from build123d import *

# Parameters (mm, degrees)
BOSS_EXTRUDE1_DEPTH     = 6.1
SKETCH3_R               = 1.25
CUT_EXTRUDE1_DEPTH      = 28.622092607
MIRROR1_COPY_1_SKETCH_R = 1.25
MIRROR1_COPY_1_DEPTH    = 28.622092607
FILLET1_R               = 1


with BuildPart() as part:
    # Sketch1 → Boss-Extrude1 (new, symmetric)
    with BuildSketch(Plane.XY):
        Polygon((11.6, 7.8), (16.1, 7.8), (16.1, 6.7), (11.6, 6.7), (11.6, -13.8), (-11.6, -13.8), (-11.6, 6.7), (-16.1, 6.7), (-16.1, 7.8), (-11.6, 7.8), (-11.6, 13.8), (11.6, 13.8), align=None)
    extrude(amount=BOSS_EXTRUDE1_DEPTH, both=True)

    # Sketch2 → Revolve1 (revolve)
    with BuildSketch(Plane.XY, mode=Mode.PRIVATE) as revolve1_sk:
        Polygon((-5.6, 18.1), (-8.1, 18.1), (-8.1, 14.8), (-9.430450184, 14.8), (-9.85, 14.3), (-9.85, 13.8), (-5.6, 13.8), align=None)
    revolve(revolve1_sk.sketch.rotate(Axis((-5.6, 13.8, 0), (0, 1, 0)), 270), axis=Axis((-5.6, 13.8, 0), (0, 1, 0)))

    # Sketch3 → Cut-Extrude1 (cut, through all)
    with BuildSketch(Plane(origin=(0, 7.8, 0), x_dir=(1, 0, 0), z_dir=(0, 1, 0))):
        with Locations(Location((14.15, 3.55, 0), (0, 0, 270))):
            Circle(SKETCH3_R)
        with BuildLine():
            Line((16.1, 0), (13.1, 0))
            Line((13.1, 0), (12, 0))
            ThreePointArc((12, 0), (12.322182541, 0.777817459), (13.1, 1.1))
            Line((13.1, 1.1), (16.1, 1.1))
            Line((16.1, 1.1), (16.1, 0))
        make_face()
    cut_extrude1 = extrude(amount=-CUT_EXTRUDE1_DEPTH, mode=Mode.SUBTRACT)

    # Mirror4: Cut-Extrude1 across plane
    add(cut_extrude1.mirror(Plane(origin=(0, 0, 0), x_dir=(0, 0, 1), z_dir=(1, 0, 0))), mode=Mode.SUBTRACT)

    # Mirror1: Cut-Extrude1 across plane
    add(cut_extrude1.mirror(Plane(origin=(16.1, -13.8, 0), x_dir=(1, 0, 0), z_dir=(0, 0, 1))), mode=Mode.SUBTRACT)

    # Mirror1 copy 1 sketch → Mirror1 copy 1 (cut, through all)
    with BuildSketch(Plane(origin=(0, 7.8, 0), x_dir=(-1, 0, 0), z_dir=(0, 1, 0))):
        with Locations(Location((14.15, 3.55, 0), (0, 0, 270))):
            Circle(MIRROR1_COPY_1_SKETCH_R)
        with BuildLine():
            Line((16.1, 0), (13.1, 0))
            Line((13.1, 0), (12, 0))
            ThreePointArc((12, 0), (12.322182541, 0.777817459), (13.1, 1.1))
            Line((13.1, 1.1), (16.1, 1.1))
            Line((16.1, 1.1), (16.1, 0))
        make_face()
    extrude(amount=-MIRROR1_COPY_1_DEPTH, mode=Mode.SUBTRACT)

    # Fillet1
    fillet1_edges = [part.edges().sort_by_distance(p)[0] for p in [
        (-16.1, 7.25, 6.1),
        (16.1, 7.25, -6.1),
        (-16.1, 7.25, -6.1),
        (16.1, 7.25, 6.1),
    ]]
    fillet(fillet1_edges, radius=FILLET1_R)


solid = part.part
Check sheet for the modelled part. Datum: model origin and axes. Units: mm. A direction names the side the tool comes from. Coordinates: 2 decimals unless noted, no trailing zeros. Write each loop counter-clockwise with the first axis right and the second up, starting at its lowest first coordinate (ties: lowest second). Pieces come first, ordered by that corner, then holes.
Item 1: Cross-section at A-A on x = 14.15. Record the boundary of the cut face in (y, z), then the cut area to 3 significant figures.
Numbers:
outline: (6.7, -6.1) - (7.8, -6.1) - (7.8, -4.8) - (6.7, -4.8) - close; (6.7, -2.3) - (7.8, -2.3) - (7.8, -1.1) - (6.7, -1.1) - close; (6.7, 1.1) - (7.8, 1.1) - (7.8, 2.3) - (6.7, 2.3) - close; (6.7, 4.8) - (7.8, 4.8) - (7.8, 6.1) - (6.7, 6.1) - close
area: 5.50 mm2
Item 2: Scan lines: probe 1 along Z at (x, y) = (-14, 7); probe 2 along X at (y, z) = (7.6, -3.55); probe 3 along Y at (x, z) = (-3.5, 1.5). Record each from-to range of solid material in increasing order.
Numbers:
probe 1: z = -6.1 to -4.79, -2.31 to -1.1, 1.1 to 2.31, 4.79 to 6.1
probe 2: x = -16.1 to -15.4, -12.9 to 12.9, 15.4 to 16.1
probe 3: y = -13.8 to 14.8
Item 3: Cross-section at B-B on x = -5.6. Record the boundary of the cut face in (y, z), then the cut area to 3 significant figures.
Numbers:
outline: (-13.8, -6.1) - (13.8, -6.1) - (13.8, -4.25) - (14.3, -4.25) - (14.8, -3.83) - (14.8, -2.5) - (18.1, -2.5) - (18.1, 2.5) - (14.8, 2.5) - (14.8, 3.83) - (14.3, 4.25) - (13.8, 4.25) - (13.8, 6.1) - (-13.8, 6.1) - close
area: 362 mm2
Item 4: Mould release check, pull along Z, two halves, no side actions. Record for faces 1 (the face through (-16.1, 7, -3)), 2 (the face through (15, 7, -1.1)), 3 (the face through (15.815, 7.242, -5.799)): released by +Z, released by -Z, zero draft, split by the parting line, or undercut.
Numbers:
face 1: zero draft
face 2: undercut
face 3: released by -Z
Item 5: Access from +Z, -Z, +X, -X, +Y, -Y to the whole of each face (thin tool, end or side, straight path). Record for faces 4 (the face through (-13.8, 6.7, 1.4)), 5 (the face through (-13.9, 7.8, 1.4)), 6 (the face through (-6, 14.8, 3)), 7 (the face through (-15, 7, -1.1)), 8 (the face through (11.6, 11, 0)).
Numbers:
face 4: +Z, -Z, -X, -Y
face 5: +Z, -Z, -X, +Y
face 6: +Y
face 7: -X, +Y, -Y
face 8: +Z, -Z, +X, +Y
Item 6: Cross-section at D-D on z = -3. Count the separate pieces of the cut face and the enclosed holes in it, then the cut area to 3 significant figures.
Numbers:
separate pieces: 3
enclosed holes: 0
area: 651 mm2
Item 7: Depth check by flat-ended pin: pin 1 Ø6.5 at (y, z) = (9.5, -3) entering from -X; pin 2 Ø1 at (y, z) = (-4, -1) entering from -X; pin 3 Ø5 at (x, z) = (-13, 3) entering from +Y; pin 4 Ø3.5 at (x, z) = (-14.5, 2.5) entering from -Y. Enter the tip coordinate at first touch or a pass-through.
Numbers:
pin 1: stops at x = -16.1
pin 2: stops at x = -11.6
pin 3: stops at y = 13.8
pin 4: stops at y = 6.7
Item 8: Cross-section at C-C on y = -3. Record the boundary of the cut face in (x, z), then the cut area to 3 significant figures.
Numbers:
outline: (-11.6, -6.1) - (11.6, -6.1) - (11.6, 6.1) - (-11.6, 6.1) - close
area: 283 mm2
